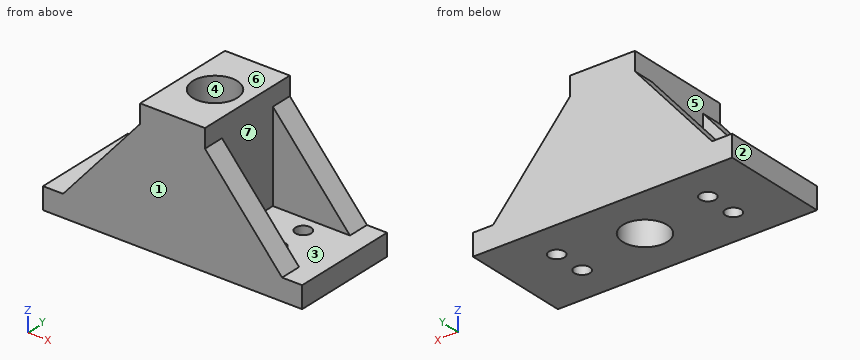
from build123d import *

# Parameters (mm, degrees)
SKETCH_1_W               = 40
SKETCH_1_H               = 15
EXTRUDE_1_DEPTH          = 5
SKETCH_2_R               = 5.15
SKETCH_2_R_2             = 1.8
CUT_EXTRUDE_1_DEPTH      = 5
SKETCH_3_W               = 15
SKETCH_3_H               = 15
SKETCH_3_R               = 5.05
EXTRUDE_2_DEPTH          = 25
SKETCH_4_R               = 5.5
CUT_EXTRUDE_2_DEPTH      = 31
SKETCH_5_W               = 10
SKETCH_5_H               = 15
EXTRUDE_3_DEPTH          = 5
SKETCH_6_R               = 1.8
CUT_EXTRUDE_3_DEPTH      = 5
SKETCH_7_W               = 60
SKETCH_7_H               = 5
EXTRUDE_4_DEPTH          = 5
SKETCH_8_W               = 15
SKETCH_8_H               = 5
EXTRUDE_5_DEPTH          = 25
RIB_1_REACH              = 51.244
SKETCH_9_WALL_W          = 127.83111072
SKETCH_9_WALL_H          = 5
MIRROR_2_COPY_1_REACH    = 51.244
MIRROR_2_COPY_1_SKETCH_W = 127.83111072
MIRROR_2_COPY_1_SKETCH_H = 5
SKETCH_11_R              = 1.8
EXTRUDE_6_DEPTH          = 5
SKETCH_12_R              = 1.8
CUT_EXTRUDE_4_DEPTH      = 5
SKETCH_13_R              = 5.5
SKETCH_13_R_2            = 5.15
EXTRUDE_7_DEPTH          = 25


with BuildPart() as part:
    # 草图1 → 凸台-拉伸1 (new body)
    with BuildSketch(Plane.XY):
        Rectangle(SKETCH_1_W, SKETCH_1_H)
    extrude(amount=EXTRUDE_1_DEPTH)

    # 草图2 → 切除-拉伸1 (cut)
    with BuildSketch(Plane.XY.offset(5)):
        Circle(SKETCH_2_R)
        with Locations((-12, 0)):
            Circle(SKETCH_2_R_2)
        with Locations(Location((12, 0, 0), (0, 0, 180))):
            Circle(SKETCH_2_R_2)
    extrude(amount=-CUT_EXTRUDE_1_DEPTH, mode=Mode.SUBTRACT)

    # 草图3 → 凸台-拉伸2 (add)
    with BuildSketch(Plane.XY.offset(5)):
        Rectangle(SKETCH_3_W, SKETCH_3_H)
        Circle(SKETCH_3_R, mode=Mode.SUBTRACT)
    extrude(amount=EXTRUDE_2_DEPTH)

    # 草图4 → 切除-拉伸2 (cut)
    with BuildSketch(Plane(origin=(0, 0, 5), x_dir=(-1, 0, 0), z_dir=(0, 0, -1))):
        Circle(SKETCH_4_R)
    extrude(amount=-CUT_EXTRUDE_2_DEPTH, mode=Mode.SUBTRACT)

    # 草图5 → 凸台-拉伸3 (add)
    with BuildSketch(Plane.XY.offset(5)):
        with Locations((-25, 0)):
            Rectangle(SKETCH_5_W, SKETCH_5_H)
        with Locations((25, 0)):
            Rectangle(SKETCH_5_W, SKETCH_5_H)
    extrude(amount=-EXTRUDE_3_DEPTH)

    # 草图6 → 切除-拉伸3 (cut)
    with BuildSketch(Plane.XY.offset(5)):
        with Locations((-24, 0)):
            Circle(SKETCH_6_R)
        with Locations(Location((24, 0, 0), (0, 0, 180))):
            Circle(SKETCH_6_R)
    extrude(amount=-CUT_EXTRUDE_3_DEPTH, mode=Mode.SUBTRACT)

    # 草图7 → 凸台-拉伸4 (add)
    with BuildSketch(Plane.XY.offset(5)):
        with Locations((0, 10)):
            Rectangle(SKETCH_7_W, SKETCH_7_H)
        with Locations((0, -10)):
            Rectangle(SKETCH_7_W, SKETCH_7_H)
    extrude(amount=-EXTRUDE_4_DEPTH)

    # 草图8 → 凸台-拉伸5 (add)
    with BuildSketch(Plane.XY.offset(5)):
        with Locations((0, 10)):
            Rectangle(SKETCH_8_W, SKETCH_8_H)
        with Locations((0, -10)):
            Rectangle(SKETCH_8_W, SKETCH_8_H)
    extrude(amount=EXTRUDE_5_DEPTH)

    # 草图9 wall → 筋1 (add, up to next)
    with BuildSketch(Plane(origin=(-16.427615827, 12.5, 15.353801199), x_dir=(0.653020400469, 0, 0.75734031754), z_dir=(0.75734031754, 0, -0.653020400469)), mode=Mode.PRIVATE) as rib_1_sk1:
        with Locations((0, 2.5)):
            Rectangle(SKETCH_9_WALL_W, SKETCH_9_WALL_H)
    rib_1_tool1 = extrude(rib_1_sk1.sketch, amount=RIB_1_REACH, mode=Mode.PRIVATE) - part.part
    rib_1 = rib_1_tool1.solids().sort_by_distance((-16.427615827, 12.5, 15.353801199))[0]
    add(rib_1)

    # 镜向1: 筋1 across plane
    add(rib_1.mirror(Plane.ZX))

    # 镜向2: 筋1 across plane
    add(rib_1.mirror(Plane.ZY))

    # 镜向2 copy 1 sketch → 镜向2 copy 1 (add, up to next)
    with BuildSketch(Plane(origin=(16.427615827, -12.5, 15.353801199), x_dir=(-0.653020400469, 0, 0.75734031754), z_dir=(-0.75734031754, 0, -0.653020400469)), mode=Mode.PRIVATE) as mirror_2_copy_1_sk1:
        with Locations((0, 2.5)):
            Rectangle(MIRROR_2_COPY_1_SKETCH_W, MIRROR_2_COPY_1_SKETCH_H)
    mirror_2_copy_1_tool1 = extrude(mirror_2_copy_1_sk1.sketch, amount=MIRROR_2_COPY_1_REACH, mode=Mode.PRIVATE) - part.part
    add(mirror_2_copy_1_tool1.solids().sort_by_distance((16.427615827, -12.5, 15.353801199))[0])

    # 草图11 → 凸台-拉伸6 (add)
    with BuildSketch(Plane.XY.offset(5)):
        with Locations((-24, 0)):
            Circle(SKETCH_11_R)
        with Locations((-12, 0)):
            Circle(SKETCH_11_R)
        with Locations((12, 0)):
            Circle(SKETCH_11_R)
        with Locations((24, 0)):
            Circle(SKETCH_11_R)
    extrude(amount=-EXTRUDE_6_DEPTH)

    # 草图12 → 切除-拉伸4 (cut)
    with BuildSketch(Plane.XY.offset(5)):
        with Locations((-17.5, 3.75)):
            Circle(SKETCH_12_R)
        with Locations(Location((-17.5, -3.75, 0), (0, 0, 180))):
            Circle(SKETCH_12_R)
        with Locations((17.5, -3.75)):
            Circle(SKETCH_12_R)
        with Locations(Location((17.5, 3.75, 0), (0, 0, 180))):
            Circle(SKETCH_12_R)
    extrude(amount=-CUT_EXTRUDE_4_DEPTH, mode=Mode.SUBTRACT)

    # 草图13 → 凸台-拉伸7 (add)
    with BuildSketch(Plane.XY.offset(5)):
        Circle(SKETCH_13_R)
        Circle(SKETCH_13_R_2, mode=Mode.SUBTRACT)
    extrude(amount=EXTRUDE_7_DEPTH)


solid = part.part
Source: CAD feature listing. Evaluate the final solid. Frame: model axes, mm. Face numbers are marked on the shaded views. A direction names the side the tool comes from. Round coordinates to 2 decimals unless told otherwise and drop trailing zeros. Loops run counter-clockwise (first coordinate to the right, second up) from the corner with the lowest first, then second, coordinate; pieces in that order, holes last. Notation, with made-up numbers: (-4.5, 85.5) - (48.5, 85.5) arc R31 cw to (48.5, 109.5) - close; hole circle Ø11 at (87, 62). An arc over 180 degrees is marked (long way). Write item = value, one per line. Start each with the question number.
Item 1: First-contact query: pin 1 Ø2 at (x, y) = (-17.5, 3.75) entering from -Z; pin 2 Ø10 at (y, z) = (9.5, 20) entering from +X; pin 3 Ø6 at (x, y) = (17.5, -3.75) entering from +Z; pin 4 Ø2 at (x, y) = (21.5, 8) entering from +Z. Flat tips, straight axial feed; report the tip coordinate or a pass-through.
Item 2: Material intervals for line 1 (Y direction, x = -17.5, z = 3.65); line 2 (Y direction, x = -8.5, z = 20); line 3 (X direction, y = 3.5, z = 2.5), sorted ascending.
Item 3: Reachability of the marked faces 5, 6 and 7 from +Z, -Z, +X, -X, +Y, -Y: full face, straight path, thin tool, end or side. Return the list, or none.
Item 4: Section query C-C on y = 3.75. Output: boundary loops of the cut face in (x, z), plus the area to 3 significant figures.
Item 5: Section query D-D on z = 15. Output: boundary loops of the cut face in (x, y), plus the area to 3 significant figures.
Item 6: Mould query, pull axis Y, two halves, no side actions, for the marked faces 1, 2, 3 and 4. Classes: released by +Y, released by -Y, zero draft, split by the parting line, or undercut.
Item 7: Section query B-B on x = 0. Output: boundary loops of the cut face in (y, z).
Item 8: Section query A-A on y = 0. Output: boundary loops of the cut face in (x, z), plus the area to 3 significant figures.
Results list:
q1.pin_1 = through
q1.pin_2 = 16.73
q1.pin_3 = 5
q1.pin_4 = 10.63
q2.line_1 = -12.5 to -5.55, -1.95 to 1.95, 5.55 to 12.5
q2.line_2 = -12.5 to -7.5, 7.5 to 12.5
q2.line_3 = -30 to -19.28, -15.72 to -3.78, 3.78 to 15.72, 19.28 to 30
q3.face_5 = +Z, -X
q3.face_6 = +Z, +X, -X, +Y, -Y
q3.face_7 = +Z, +X
q4.outline = (-30, 0) - (-19.3, 0) - (-19.3, 5) - (-30, 5) - close; (-15.7, 0) - (-3.53, 0) - (-3.53, 30) - (-7.5, 30) - (-7.5, 5) - (-15.7, 5) - close; (3.53, 0) - (15.7, 0) - (15.7, 5) - (7.5, 5) - (7.5, 30) - (3.53, 30) - close; (19.3, 0) - (30, 0) - (30, 5) - (19.3, 5) - close
q4.area = 427 mm²
q5.outline = (-16.73, -12.5) - (16.73, -12.5) - (16.73, -7.5) - (7.5, -7.5) - (7.5, 7.5) - (16.73, 7.5) - (16.73, 12.5) - (-16.73, 12.5) - (-16.73, 7.5) - (-7.5, 7.5) - (-7.5, -7.5) - (-16.73, -7.5) - close; hole circle Ø10.3 at (0, 0)
q5.area = 476 mm²
q6.face_1 = released by -Y
q6.face_2 = zero draft
q6.face_3 = undercut
q6.face_4 = undercut
q7.outline = (-12.5, 0) - (-5.15, 0) - (-5.15, 30) - (-12.5, 30) - close; (5.15, 0) - (12.5, 0) - (12.5, 30) - (5.15, 30) - close
q8.outline = (-30, 0) - (-5.15, 0) - (-5.15, 30) - (-7.5, 30) - (-7.5, 5) - (-30, 5) - close; (5.15, 0) - (30, 0) - (30, 5) - (7.5, 5) - (7.5, 30) - (5.15, 30) - close
q8.area = 366 mm²
